Check sheet for the modelled part. Datum: model origin and axes. Units: mm. A direction names the side the tool comes from. Round coordinates to 2 decimals unless told otherwise and drop trailing zeros. Write each loop counter-clockwise with the first axis right and the second up, starting at its lowest first coordinate (ties: lowest second). Pieces come first, ordered by that corner, then holes. Notation, with made-up numbers: (-36, -17.75) - (-5, -17.75) arc R25 cw to (-5, 7.25) - close; hole circle Ø3 at (-9.5, 89). An arc over 180 degrees is marked (long way). Use one line per item in the form item = value. Start each with the question number.
1) Draft check along Y on faces 5 (the face through (-4.93, 9.73, 28.99)), 6 (the face through (82, 20, 19)), 7 (the face through (38, 69.2, 29)). Enter one of: +Y half, -Y half, draft (parallel to the pull), parting line (faces both ways), or undercut.
2) Section check C-C (y = 14.5). Record the boundary of the cut face in (x, z), then the cut area to 3 significant figures.
3) Section check B-B (x = 21.5). Record the boundary of the cut face in (y, z), then the cut area to 3 significant figures.
4) Section check A-A (z = 25). Record the boundary of the cut face in (x, y).
5) Gauge pin test, flat ends, axial feed: P1, Ø3, axis at y = 8.5, z = 5.5, coming from the -X side; P2, Ø20, axis at x = 20, y = 36.5, coming from the +Z side; P3, Ø1.6, axis at x = -7, z = 29, coming from the -Y side; P4, Ø10, axis at x = 65.5, y = 51.5, coming from the -Z side. Record the tip position at first contact, or that the pin passes through.
6) Scan lines: probe 1 along Y at (x, z) = (53, 6); probe 2 along X at (y, z) = (29.5, 18.5); probe 3 along Z at (x, y) = (67, 18.5). Record each from-to range of solid material in increasing order.
7) Section check D-D (z = 4.75). Record the boundary of the cut face in (x, y), then the cut area to 3 significant figures.
8) Set-up check for faces 1 (the face through (37, 0.8, 29)), 2 (the face through (79.93, 60.27, 28.99)), 3 (the face through (-4.81, 60.52, 28.99)), 4 (the face through (-7, 20, 19)): record each of +Z, -Z, +X, -X, +Y, -Y from which the full face is reachable in a straight line by a thin tool's end or side.
from build123d import *
from build123d.topology import SkipClean

# Parameters (mm, degrees)
BOSS_EXTRUDE4_DEPTH  = 10
BOSS_EXTRUDE10_DEPTH = 18
BOSS_EXTRUDE11_DEPTH = 2
CUT_EXTRUDE8_DEPTH   = 28


with BuildPart() as part:
    # Sketch1 → Boss-Extrude4 (new body)
    with BuildSketch(Plane.XY):
        with BuildLine():
            Line((0, 0), (75, 0))
            ThreePointArc((75, 0), (86.502118606, 35), (75, 70))
            Line((75, 70), (0, 70))
            ThreePointArc((0, 70), (-11.502118606, 35), (0, 0))
        make_face()
    extrude(amount=BOSS_EXTRUDE4_DEPTH)

    # Sketch4 → Boss-Extrude10 (add)
    with SkipClean():  # the faces are left unmerged after this step: merging them gives an invalid solid
        with BuildSketch(Plane.XY.offset(10)):
            with BuildLine():
                Line((79.502118606, 20), (84.563561053, 20))
                ThreePointArc((84.563561053, 20), (80.729546072, 9.546799317), (75, 0))
                Line((75, 0), (0, 0))
                ThreePointArc((0, 0), (-5.729546072, 9.546799317), (-9.563561053, 20))
                Line((-9.563561053, 20), (-4.502118606, 20))
                Line((-4.502118606, 20), (-4.502118606, 50))
                Line((-4.502118606, 50), (-9.563561053, 50))
                ThreePointArc((-9.563561053, 50), (-5.729546072, 60.453200683), (0, 70))
                Line((0, 70), (75, 70))
                ThreePointArc((75, 70), (80.729546072, 60.453200683), (84.563561053, 50))
                Line((84.563561053, 50), (79.502118606, 50))
                Line((79.502118606, 50), (79.502118606, 20))
            make_face()
        extrude(amount=BOSS_EXTRUDE10_DEPTH)

    # Sketch9 → Boss-Extrude11 (add)
    with SkipClean():  # the faces are left unmerged after this step: merging them gives an invalid solid
        with BuildSketch(Plane.XY.offset(28)):
            with BuildLine():
                Line((-8.516485165, 50.8), (-3.702118606, 50.8))
                Line((-3.702118606, 50.8), (-3.702118606, 19.2))
                Line((-3.702118606, 19.2), (-8.516485165, 19.2))
                ThreePointArc((-8.516485165, 19.2), (-4.869685973, 9.605067408), (0.405981163, 0.8))
                Line((0.405981163, 0.8), (74.594018837, 0.8))
                ThreePointArc((74.594018837, 0.8), (79.869685973, 9.605067408), (83.516485165, 19.2))
                Line((83.516485165, 19.2), (78.702118606, 19.2))
                Line((78.702118606, 19.2), (78.702118606, 50.8))
                Line((78.702118606, 50.8), (83.516485165, 50.8))
                ThreePointArc((83.516485165, 50.8), (79.869685973, 60.394932592), (74.594018837, 69.2))
                Line((74.594018837, 69.2), (0.405981163, 69.2))
                ThreePointArc((0.405981163, 69.2), (-4.869685973, 60.394932592), (-8.516485165, 50.8))
            make_face()
        extrude(amount=BOSS_EXTRUDE11_DEPTH)

    # Sketch10 → Cut-Extrude8 (cut)
    with SkipClean():  # the faces are left unmerged after this step: merging them gives an invalid solid
        with BuildSketch(Plane.XY.offset(30)):
            with BuildLine():
                Line((-6.908101654, 52), (-2.502118606, 52))
                Line((-2.502118606, 52), (-2.502118606, 18))
                Line((-2.502118606, 18), (-6.908101654, 18))
                ThreePointArc((-6.908101654, 18), (-3.68947636, 9.922539293), (0.720250379, 2.428593046))
                ThreePointArc((0.720250379, 2.428593046), (1.077995513, 2.113600837), (1.540917238, 2))
                Line((1.540917238, 2), (73.459082762, 2))
                ThreePointArc((73.459082762, 2), (73.922004487, 2.113600837), (74.279749621, 2.428593046))
                ThreePointArc((74.279749621, 2.428593046), (78.68947636, 9.922539293), (81.908101654, 18))
                Line((81.908101654, 18), (77.502118606, 18))
                Line((77.502118606, 18), (77.502118606, 52))
                Line((77.502118606, 52), (81.908101654, 52))
                ThreePointArc((81.908101654, 52), (78.68947636, 60.077460707), (74.279749621, 67.571406954))
                ThreePointArc((74.279749621, 67.571406954), (73.922004487, 67.886399163), (73.459082762, 68))
                Line((73.459082762, 68), (1.540917238, 68))
                ThreePointArc((1.540917238, 68), (1.077995513, 67.886399163), (0.720250379, 67.571406954))
                ThreePointArc((0.720250379, 67.571406954), (-3.68947636, 60.077460707), (-6.908101654, 52))
            make_face()
        extrude(amount=-CUT_EXTRUDE8_DEPTH, mode=Mode.SUBTRACT)


solid = part.part
Results are:
q1.face_5 = -Y half
q1.face_6 = undercut
q1.face_7 = +Y half
q2.outline = (-7.83, 0) - (82.83, 0) - (82.83, 28) - (81.97, 28) - (81.97, 30) - (80.69, 30) - (80.69, 2) - (-5.69, 2) - (-5.69, 30) - (-6.97, 30) - (-6.97, 28) - (-7.83, 28) - close
q2.area = 298 mm²
q3.outline = (0, 0) - (70, 0) - (70, 28) - (69.2, 28) - (69.2, 30) - (68, 30) - (68, 2) - (2, 2) - (2, 30) - (0.8, 30) - (0.8, 28) - (0, 28) - close
q3.area = 249 mm²
q4.outline = (-9.56, 20) arc R59 ccw to (0, 0) - (75, 0) arc R59 ccw to (84.56, 20) - (79.5, 20) - (79.5, 50) - (84.56, 50) arc R59 ccw to (75, 70) - (0, 70) arc R59 ccw to (-9.56, 50) - (-4.5, 50) - (-4.5, 20) - close; hole (-6.91, 18) arc R57 ccw to (0.72, 2.43) arc R1 ccw to (1.54, 2) - (73.46, 2) arc R1 ccw to (74.28, 2.43) arc R57 ccw to (81.91, 18) - (77.5, 18) - (77.5, 52) - (81.91, 52) arc R57 ccw to (74.28, 67.57) arc R1 ccw to (73.46, 68) - (1.54, 68) arc R1 ccw to (0.72, 67.57) arc R57 ccw to (-6.91, 52) - (-2.5, 52) - (-2.5, 18) - close
q5.P1 = -5.94
q5.P2 = 2
q5.P3 = 12.55
q5.P4 = 0
q6.probe_1 = 0 to 2, 68 to 70
q6.probe_2 = -4.5 to -2.5, 77.5 to 79.5
q6.probe_3 = 0 to 2
q7.outline = (0, 0) - (75, 0) arc R59 ccw to (75, 70) - (0, 70) arc R59 ccw to start; hole (-6.91, 18) arc R57 ccw to (0.72, 2.43) arc R1 ccw to (1.54, 2) - (73.46, 2) arc R1 ccw to (74.28, 2.43) arc R57 ccw to (81.91, 18) - (77.5, 18) - (77.5, 52) - (81.91, 52) arc R57 ccw to (74.28, 67.57) arc R1 ccw to (73.46, 68) - (1.54, 68) arc R1 ccw to (0.72, 67.57) arc R57 ccw to (-6.91, 52) - (-2.5, 52) - (-2.5, 18) - close
q7.area = 1,000 mm²
q8.face_1 = +Z, +X, -X, -Y
q8.face_2 = +Z, +X, +Y
q8.face_3 = +Z, -X, +Y
q8.face_4 = +Z, -X
